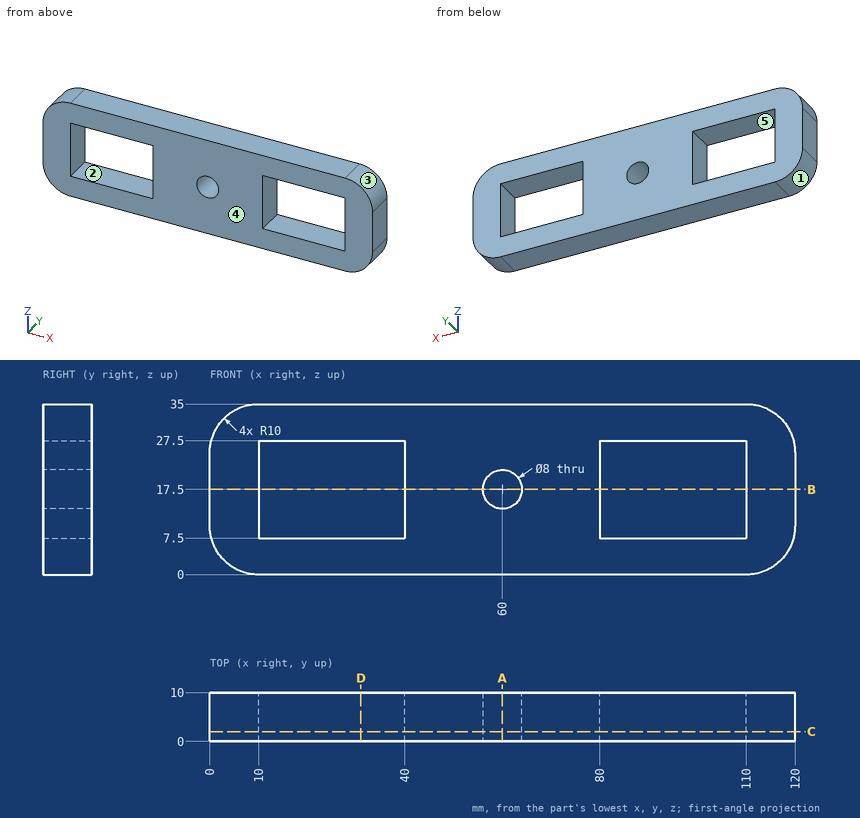
The drawing under review shows one solid part. Ordinate dimensions are in mm from its lowest x, y, z. A direction names the side the tool comes from. Coordinates: 2 decimals unless noted, no trailing zeros. Write each loop counter-clockwise with the first axis right and the second up, starting at its lowest first coordinate (ties: lowest second). Pieces come first, ordered by that corner, then holes. Notation, with made-up numbers: (55.25, -20) -> (96.25, -20) arc R17 ccw to (96.25, 13) -> close; hole circle Ø4 at (13, -21.5). An arc over 180 degrees is marked (long way). One line per item, written item: value. Start each with the question number.
Q1. Clearance check with a flat-ended pin moving along its axis: P1, Ø4, axis at y = 1.5, z = 28.5, coming from the -X side. State where the tip first meets the part, or that it passes through.
Q2. Add section C-C, the plane y = 2. Give the boundary of the cut face in (x, z).
Q3. To check wall thickness, follow probe 1 along X at (y, z) = (3.5, 17.5); probe 2 along X at (y, z) = (4.75, 22); probe 3 along Z at (x, y) = (60, 2.5). State the ranges of each line that lie inside material, in increasing order.
Q4. Add section B-B, the plane z = 17.5. Give the boundary of the cut face in (x, y), then the cut area to 3 significant figures.
Q5. Add section D-D, the plane x = 31. Give the boundary of the cut face in (y, z).
Q6. For the marked faces 4 and 5, list the 3-axis set-ups (+Z, -Z, +X, -X, +Y, -Y) from which the entire face can be reached by the end or side of a thin tool; tool diameter is ignored.
Q7. The part is to be moulded in two halves that separate along Z. For the marked faces 1, 2 and 3, say which applies: +Z half, -Z half, draft (parallel to the pull), parting line (faces both ways), or undercut.
Q8. Add section A-A, the plane x = 60. Give the boundary of the cut face in (y, z).
Response:
1. P1: x = 0.11
2. outline: (0, 10) arc R10 ccw to (10, 0) -> (110, 0) arc R10 ccw to (120, 10) -> (120, 25) arc R10 ccw to (110, 35) -> (10, 35) arc R10 ccw to (0, 25) -> close; hole (10, 7.5) -> (40, 7.5) -> (40, 27.5) -> (10, 27.5) -> close; hole circle Ø8 at (60, 17.5); hole (80, 7.5) -> (110, 7.5) -> (110, 27.5) -> (80, 27.5) -> close
3. probe 1: 0 to 10, 40 to 56, 64 to 80, 110 to 120
3. probe 2: 0 to 10, 40 to 80, 110 to 120
3. probe 3: 0 to 13.5, 21.5 to 35
4. outline: (0, 0) -> (10, 0) -> (10, 10) -> (0, 10) -> close; (40, 0) -> (56, 0) -> (56, 10) -> (40, 10) -> close; (64, 0) -> (80, 0) -> (80, 10) -> (64, 10) -> close; (110, 0) -> (120, 0) -> (120, 10) -> (110, 10) -> close
4. area: 520 mm²
5. outline: (0, 0) -> (10, 0) -> (10, 7.5) -> (0, 7.5) -> close; (0, 27.5) -> (10, 27.5) -> (10, 35) -> (0, 35) -> close
6. face 4: +Z, -Z, +X, -X, -Y
6. face 5: +Y, -Y
7. face 1: -Z half
7. face 2: undercut
7. face 3: +Z half
8. outline: (0, 0) -> (10, 0) -> (10, 13.5) -> (0, 13.5) -> close; (0, 21.5) -> (10, 21.5) -> (10, 35) -> (0, 35) -> close
